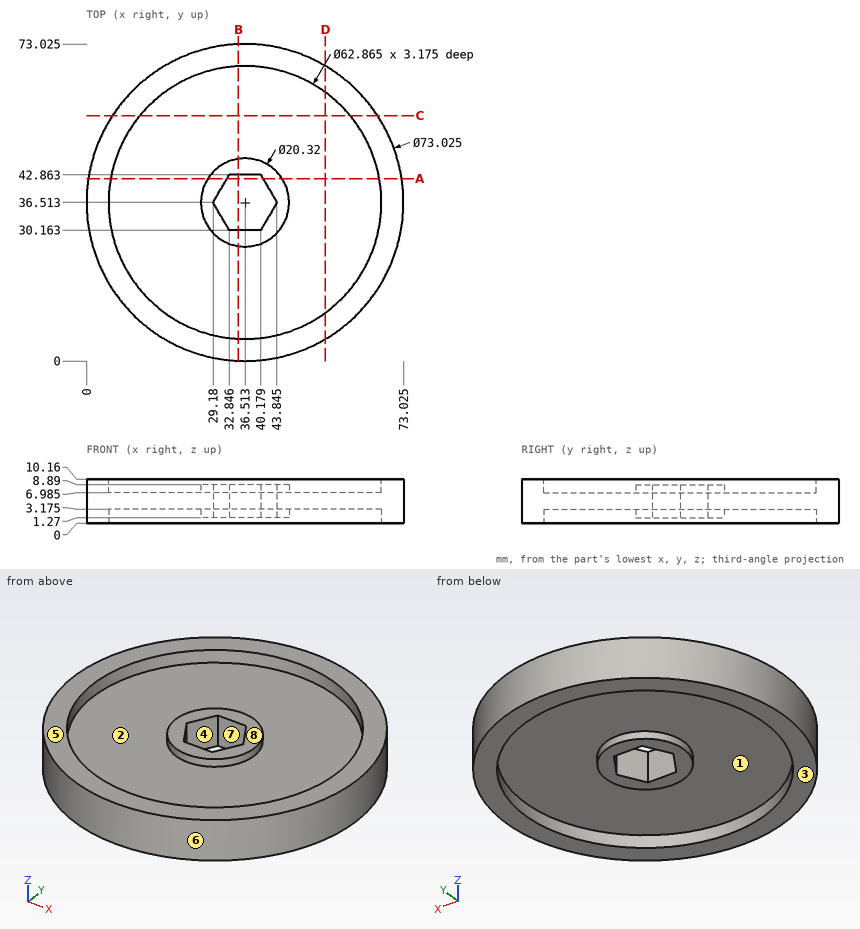
Print and shaded views of the part. All mm, measured from the part's lowest x, y and z. A direction names the side the tool comes from. Coordinates: 2 decimals unless noted, no trailing zeros. Write each loop counter-clockwise with the first axis right and the second up, starting at its lowest first coordinate (ties: lowest second). Pieces come first, ordered by that corner, then holes. Notation, with made-up numbers: (14.25, 58) - (70.25, 58) arc R14 cw to (70.25, 68) - close; hole circle Ø5 at (82.25, -3.75). An arc over 180 degrees is marked (long way). One line per question, with ' | ' between items. Start each with the question number.
Q1. Drill centre lines: line 1 (Y direction, x = 39, z = 7.5) (1 decimal); line 2 (Z direction, x = 15.5, y = 24) (1 decimal); line 3 (Y direction, x = 47, z = 2.25) (1 decimal). Where is each one in solid material? Low to high. Write a range as [from, to].
Q2. Cut at C-C, the plane y = 56.5. List the corners of the cut face in (x, z) (1 decimal).
Q3. Cut at B-B, the plane x = 35. List the corners of the cut face in (y, z) (1 decimal).
Q4. Pull direction X, two halves, no side cores. Call the marked faces 5, 6, 7 and 8: pulls with the +X half, pulls with the -X half, needs draft (parallel to the pull), parting line crosses it, or undercut.
Q5. Cut at D-D, the plane x = 55. List the corners of the cut face in (y, z) (1 decimal), then the cut area to 3 significant figures.
Q6. 3-axis set-ups, long thin cutter, end or side, ignore diameter. For the marked faces 1, 2, 3 and 4: which of +Z, -Z, +X, -X, +Y, -Y reach the whole face in a straight line?
Q7. Pin check, flat tips, straight feed: pin 1 (19 mm diameter, centred on x = 29, y = 49.5, fed in from +Z); pin 2 (6 mm diameter, centred on y = 55, z = 8.5, fed in from -X); pin 3 (6 mm diameter, centred on y = 20.5, z = 3.5, fed in from -X). Stop position of each tip, or through.
Q8. Cut at A-A, the plane y = 42. List the corners of the cut face in (x, z) (1 decimal).
Answer below:
1) line 1: [0.1, 5.2], [26.7, 30.2], [42.9, 46.4], [67.8, 72.9] | line 2: [3.2, 7] | line 3: [1.5, 6.9], [66.1, 71.5]
2) outline: (6, 0) - (12.3, 0) - (12.3, 3.2) - (60.8, 3.2) - (60.8, 0) - (67.1, 0) - (67.1, 10.2) - (60.8, 10.2) - (60.8, 7) - (12.3, 7) - (12.3, 10.2) - (6, 10.2) - close
3) outline: (0, 0) - (5.1, 0) - (5.1, 3.2) - (26.5, 3.2) - (26.5, 1.3) - (30.2, 1.3) - (30.2, 8.9) - (26.5, 8.9) - (26.5, 7) - (5.1, 7) - (5.1, 10.2) - (0, 10.2) - close; (42.9, 1.3) - (46.6, 1.3) - (46.6, 3.2) - (67.9, 3.2) - (67.9, 0) - (73, 0) - (73, 10.2) - (67.9, 10.2) - (67.9, 7) - (46.6, 7) - (46.6, 8.9) - (42.9, 8.9) - close
4) face 5: needs draft | face 6: parting line crosses it | face 7: undercut | face 8: undercut
5) outline: (5, 0) - (11.1, 0) - (11.1, 3.2) - (61.9, 3.2) - (61.9, 0) - (68, 0) - (68, 10.2) - (61.9, 10.2) - (61.9, 7) - (11.1, 7) - (11.1, 10.2) - (5, 10.2) - close | area: 317 mm^2
6) face 1: -Z | face 2: +Z | face 3: -Z, +X, -X, +Y, -Y | face 4: +Z, -Z
7) pin 1: z = 8.89 | pin 2: x = 3.45 | pin 3: x = 2.4
8) outline: (0.4, 0) - (5.6, 0) - (5.6, 3.2) - (28, 3.2) - (28, 1.3) - (32.3, 1.3) - (32.3, 8.9) - (28, 8.9) - (28, 7) - (5.6, 7) - (5.6, 10.2) - (0.4, 10.2) - close; (40.7, 1.3) - (45.1, 1.3) - (45.1, 3.2) - (67.5, 3.2) - (67.5, 0) - (72.6, 0) - (72.6, 10.2) - (67.5, 10.2) - (67.5, 7) - (45.1, 7) - (45.1, 8.9) - (40.7, 8.9) - close
